Verification items for the finished model (mm, model axes). Give positions to 0.01 mm unless a question says otherwise; leave off trailing zeros. Loops run counter-clockwise (first coordinate to the right, second up) from the corner with the lowest first, then second, coordinate; pieces in that order, holes last. Notation, with made-up numbers: (-32.75, 24) - (-16.75, 24) arc R22 cw to (-16.75, 45) - close; hole circle Ø5 at (-22.5, -21). An arc over 180 degrees is marked (long way). Answer in a Markdown table with one row per item.
Autodesk Inventor part; units mm, degrees
ref_plane "YZ Plane" through (0, 0, 0) normal (1, 0, 0) x (0, 1, 0)
ref_plane "XZ Plane" through (0, 0, 0) normal (0, 1, 0) x (-1, 0, 0)
ref_plane "XY Plane" through (0, 0, 0) normal (0, 0, 1) x (1, 0, 0)
sketch "Sketch1" plane through (0, 0, 0) normal (0, 0, 1) x (1, 0, 0)
  line L0 (-20, 12.5) -> (25, 12.5)
  line L1 (25, 12.5) -> (25, -12.5)
  line L2 (25, -12.5) -> (-20, -12.5)
  line L3 (-25, -7.5) -> (-25, 7.5)
  arc A0 (-20, 12.5) -> (-25, 7.5) centre (-20, 7.5) ccw
  arc A1 (-25, -7.5) -> (-20, -12.5) centre (-20, -7.5) ccw
  point P0 (0, 0)
  point P1 (-25, 12.5)
  point P2 (-25, -12.5)
  dimension "d0" = 25
  dimension "d1" = 50
  dimension "d2" = 5
  dimension "d5" = 12.5
  dimension "d6" = 25
extrude "Extrusion1" add sketch "Sketch1" along normal blind 5
sketch "Sketch2" plane through (0, 0, 5) normal (0, 0, 1) x (1, 0, 0)
  arc A0 (-20, 12.5) -> (-25, 7.5) centre (-20, 7.5) ccw
  arc A1 (-25, -7.5) -> (-20, -12.5) centre (-20, -7.5) ccw
  point P0 (0, 0)
hole "Hole1" at (-20, 7.5, 5) at (-20, -7.5, 5) direction (0, 0, -1) diameter 5 end through all
properties part number "DedoV2" material "MDF Medium Density Fiberboard"
Q1. Draft check along Y on faces 1 (the face through (0, 0, 0)), 2 (the face through (-23.5, -11.07, 2.46)), 3 (the face through (2, 12.5, 2)), 4 (the face through (-22.48, 7.83, 2.46)). Enter one of: +Y half, -Y half, draft (parallel to the pull), parting line (faces both ways), or undercut.
Completed:
| item | result |
|---|---|
| face 1 | draft |
| face 2 | -Y half |
| face 3 | +Y half |
| face 4 | undercut |
Q2. Sectioned sample at A-A (z = 0.7). Record the cut outline in (x, y), and give its area (3 significant figures).
Completed:
| item | result |
|---|---|
| outline | (-25, -7.5) arc R5 ccw to (-20, -12.5) - (25, -12.5) - (25, 12.5) - (-20, 12.5) arc R5 ccw to (-25, 7.5) - close; hole circle Ø5 at (-20, -7.5); hole circle Ø5 at (-20, 7.5) |
| area | 1,200 mm^2 |
Q3. Sectioned sample at B-B (y = 8.5). Record the cut outline in (x, z).
Completed:
| item | result |
|---|---|
| outline | (-24.9, 0) - (-22.29, 0) - (-22.29, 5) - (-24.9, 5) - close; (-17.71, 0) - (25, 0) - (25, 5) - (-17.71, 5) - close |
Q4. Sectioned sample at C-C (y = -7). Record the cut outline in (x, z).
Completed:
| item | result |
|---|---|
| outline | (-25, 0) - (-22.45, 0) - (-22.45, 5) - (-25, 5) - close; (-17.55, 0) - (25, 0) - (25, 5) - (-17.55, 5) - close |
Q5. Thickness scan on line 1 (Y direction, x = -20, z = 1.8); line 2 (X direction, y = 7.5, z = 2.75); line 3 (Y direction, x = -22, z = 2.8). Record the ranges inside material, lowest first.
Completed:
| item | result |
|---|---|
| line 1 | -12.5 to -10, -5 to 5, 10 to 12.5 |
| line 2 | -25 to -22.5, -17.5 to 25 |
| line 3 | -12.08 to -9, -6 to 6, 9 to 12.08 |
